from build123d import *

# Parameters (mm, degrees)
SKETCH_1_W          = 25
SKETCH_1_H          = 40
SKETCH_1_W_2        = 23
SKETCH_1_H_2        = 38
EXTRUDE_1_DEPTH     = 12.5
SKETCH_2_R          = 1.25
CUT_EXTRUDE_1_DEPTH = 10
SKETCH_3_R          = 1.5
CUT_EXTRUDE_2_DEPTH = 10


with BuildPart() as part:
    # 草图1 → 凸台-拉伸1 (new, symmetric)
    with BuildSketch(Plane.XY):
        Rectangle(SKETCH_1_W, SKETCH_1_H)
        Rectangle(SKETCH_1_W_2, SKETCH_1_H_2, mode=Mode.SUBTRACT)
    extrude(amount=EXTRUDE_1_DEPTH, both=True)

    # 草图2 → 切除-拉伸1 (cut)
    with BuildSketch(Plane(origin=(0, -19, 0), x_dir=(1, 0, 0), z_dir=(0, 1, 0))):
        with Locations(Location((7.071067812, -7.071067812, 0), (0, 0, 270))):
            Circle(SKETCH_2_R)
        with Locations(Location((7.071067812, 7.071067812, 0), (0, 0, 270))):
            Circle(SKETCH_2_R)
        with Locations(Location((-7.071067812, 7.071067812, 0), (0, 0, 270))):
            Circle(SKETCH_2_R)
        with Locations(Location((-7.071067812, -7.071067812, 0), (0, 0, 270))):
            Circle(SKETCH_2_R)
    extrude(amount=-CUT_EXTRUDE_1_DEPTH, mode=Mode.SUBTRACT)

    # 草图3 → 切除-拉伸2 (cut)
    with BuildSketch(Plane.ZY.offset(-11.5)):
        with Locations((4.5, -14.5)):
            Circle(SKETCH_3_R)
        with Locations((-4.5, -14.5)):
            Circle(SKETCH_3_R)
        with Locations((-4.5, -1.5)):
            Circle(SKETCH_3_R)
        with Locations((4.5, -1.5)):
            Circle(SKETCH_3_R)
    extrude(amount=-CUT_EXTRUDE_2_DEPTH, mode=Mode.SUBTRACT)


solid = part.part
Design review of the part built by this model. Coordinates are the model's own, in mm. A direction names the side the tool comes from. Give positions to 0.01 mm unless a question says otherwise; leave off trailing zeros. Loops run counter-clockwise (first coordinate to the right, second up) from the corner with the lowest first, then second, coordinate; pieces in that order, holes last. Notation, with made-up numbers: (75, 48) - (100, 48) arc R21 ccw to (100, 63) - close; hole circle Ø7 at (65.25, 84). An arc over 180 degrees is marked (long way). Write item = value, one per line.
1) Draft analysis for pull direction X (two halves, no side actions). For faces 1 (the face through (12.5, 0, 0)), 2 (the face through (11.993, -2.075, 5.886)), 3 (the face through (11.5, 0, 0)), state which applies: +X half, -X half, draft (parallel to the pull), parting line (faces both ways), or undercut.
Result sheet:
face_1 = +X half
face_2 = draft
face_3 = undercut
2) To check wall thickness, follow line 1 (Y direction, x = 12.15, z = -4.5); line 2 (Y direction, x = 8.75, z = -1.5); line 3 (X direction, y = -7, z = 2.5). State the ranges of each line that lie inside material, in increasing order.
Result sheet:
line_1 = -20 to -16, -13 to -3, 0 to 20
line_2 = -20 to -19, 19 to 20
line_3 = -12.5 to -11.5, 11.5 to 12.5
3) Take a section at A-A on z = -4.5. State the section outline as (x, y) points, and give its area (3 significant figures).
Result sheet:
outline = (-12.5, -20) - (12.5, -20) - (12.5, -16) - (11.5, -16) - (11.5, -19) - (-11.5, -19) - (-11.5, 19) - (11.5, 19) - (11.5, 0) - (12.5, 0) - (12.5, 20) - (-12.5, 20) - close; (11.5, -13) - (12.5, -13) - (12.5, -3) - (11.5, -3) - close
area = 120 mm2
4) Take a section at B-B on y = -14.5. State the section outline as (x, z) points, and give its area (3 significant figures).
Result sheet:
outline = (-12.5, -12.5) - (-11.5, -12.5) - (-11.5, 12.5) - (-12.5, 12.5) - close; (11.5, -12.5) - (12.5, -12.5) - (12.5, -6) - (11.5, -6) - close; (11.5, -3) - (12.5, -3) - (12.5, 3) - (11.5, 3) - close; (11.5, 6) - (12.5, 6) - (12.5, 12.5) - (11.5, 12.5) - close
area = 44.0 mm2
5) Clearance check with a flat-ended pin moving along its axis: pin 1 Ø2 at (x, z) = (-7.07, -7.07) entering from -Y. State where the tip first meets the part, or that it passes through.
Result sheet:
pin_1 = 19
6) Take a section at D-D on z = 2. State the section outline as (x, y) points.
Result sheet:
outline = (-12.5, -20) - (12.5, -20) - (12.5, 20) - (-12.5, 20) - close; hole (-11.5, -19) - (11.5, -19) - (11.5, 19) - (-11.5, 19) - close
7) Tool access review of faces 4 (the face through (12, -2.4, -5.7)), 5 (the face through (0, -20, 0)), 6 (the face through (6.31, -19.493, -8.063)), 7 (the face through (-11.5, 0, 0)), 8 (the face through (-12, 0, 12.5)): name each direction out of +Z, -Z, +X, -X, +Y, -Y from which nothing blocks a thin tool from reaching the whole face with its end or side.
Result sheet:
face_4 = +X
face_5 = +Z, -Z, +X, -X, -Y
face_6 = -Y
face_7 = +Z, -Z
face_8 = +Z, +X, -X, +Y, -Y
8) Take a section at C-C on x = 1.75. State the section outline as (y, z) points.
Result sheet:
outline = (-20, -12.5) - (-19, -12.5) - (-19, 12.5) - (-20, 12.5) - close; (19, -12.5) - (20, -12.5) - (20, 12.5) - (19, 12.5) - close
